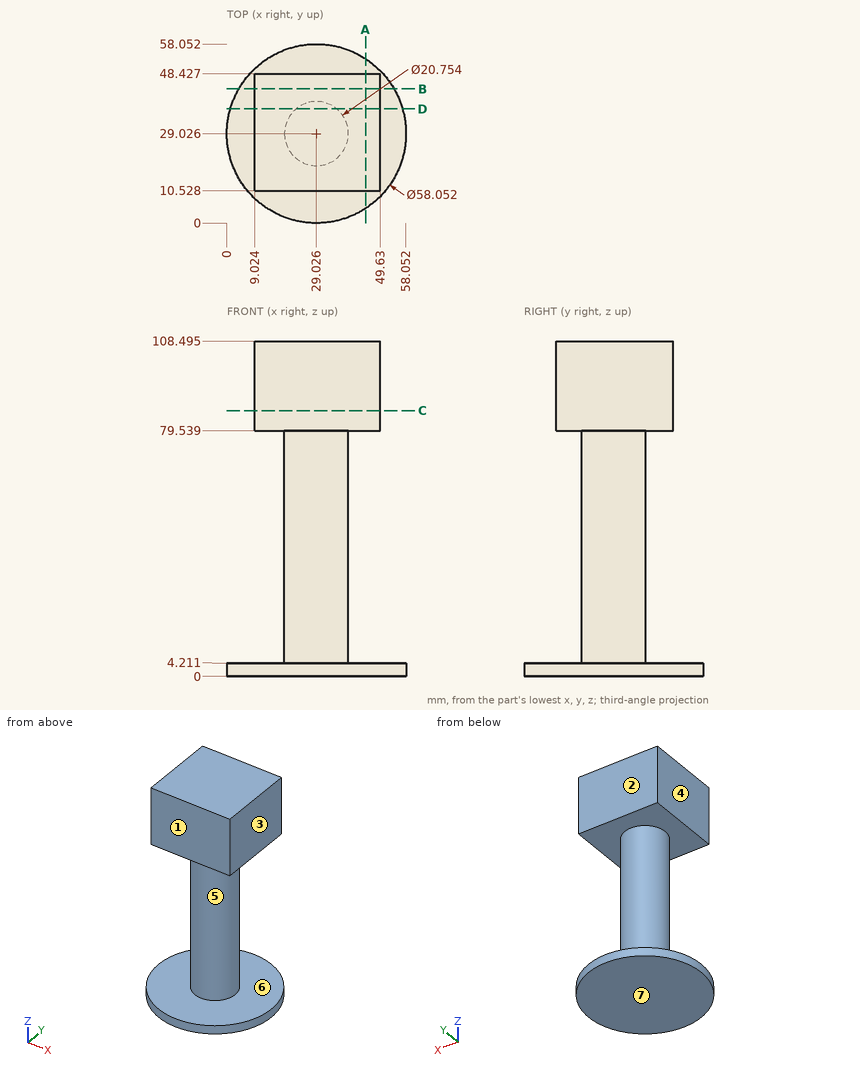
Here's the drawing with two shaded views (mm, measured from the low corner). I have some questions. A direction names the side the tool comes from. Coordinates: 2 decimals unless noted, no trailing zeros. Order: outer loops, then holes, each group sorted by start corner. A loop starts at its lowest first (then second) coordinate and runs counter-clockwise, first axis right, second up. Notation, with made-up numbers: (17.25, 20.5) -> (28.25, 20.5) arc R27 ccw to (28.25, 56.5) -> close; hole circle Ø8 at (-2, 51). An arc over 180 degrees is marked (long way). One line per question, with ' | ' between items.
Q1. I'm going to push flat-ended pins straight in: P1, Ø3, axis at x = 26.5, z = 46.5, coming from the -Y side; P2, Ø23, axis at y = 20, z = 87.5, coming from the +X side; P3, Ø8.5, axis at x = 36, z = 94, coming from the +Y side. Where does each tip first touch, or does it pass through?
Return value:
P1: y = 18.7 | P2: x = 49.63 | P3: y = 48.43
Q2. Thinking about a two-plate mould opening in Z: for the marked faces 4, 5, 6 and 7, which applies, pulls with the +Z half, pulls with the -Z half, needs draft (parallel to the pull), parting line crosses it, or undercut?
Return value:
face 4: needs draft | face 5: undercut | face 6: undercut | face 7: pulls with the -Z half
Q3. Imagine slicing it at B-B on y = 43.5. Please give me the cut outline in (x, z) (1 decimal), and give its area (3 significant figures).
Return value:
outline: (3.9, 0) -> (54.2, 0) -> (54.2, 4.2) -> (3.9, 4.2) -> close; (9, 79.5) -> (49.6, 79.5) -> (49.6, 108.5) -> (9, 108.5) -> close | area: 1,390 mm²
Q4. On a 3-axis mill with a long thin cutter (end or side, diameter ignored), from which of +Z, -Z, +X, -X, +Y, -Y can I reach the whole of each face in a straight line? I mean the marked faces 1, 2 and 3. Say none if no direction works.
Return value:
face 1: +Z, +X, -X, -Y | face 2: +Z, +X, -X, +Y | face 3: +Z, +X, +Y, -Y
Q5. Imagine slicing it at D-D on y = 37. Please give me the cut outline in (x, z) (1 decimal).
Return value:
outline: (1.1, 0) -> (56.9, 0) -> (56.9, 4.2) -> (35.7, 4.2) -> (35.7, 79.5) -> (49.6, 79.5) -> (49.6, 108.5) -> (9, 108.5) -> (9, 79.5) -> (22.4, 79.5) -> (22.4, 4.2) -> (1.1, 4.2) -> close
Q6. If I drill on L1, parallel to Z at x = 48, y = 33 (1 decimal); L2, parallel to X at y = 21, z = 99; L3, parallel to Z at x = 11, y = 48.5, over which ranges is the centre line in solid material (lowest first)?
Return value:
L1: 0 to 4.2, 79.5 to 108.5 | L2: 9.02 to 49.63 | L3: 0 to 4.21
Q7. Imagine slicing it at A-A on x = 45. Please give me the cut outline in (y, z) (1 decimal).
Return value:
outline: (4.8, 0) -> (53.3, 0) -> (53.3, 4.2) -> (4.8, 4.2) -> close; (10.5, 79.5) -> (48.4, 79.5) -> (48.4, 108.5) -> (10.5, 108.5) -> close
Q8. Imagine slicing it at C-C on z = 86. Please give me the cut outline in (x, y).
Return value:
outline: (9.02, 10.53) -> (49.63, 10.53) -> (49.63, 48.43) -> (9.02, 48.43) -> close
